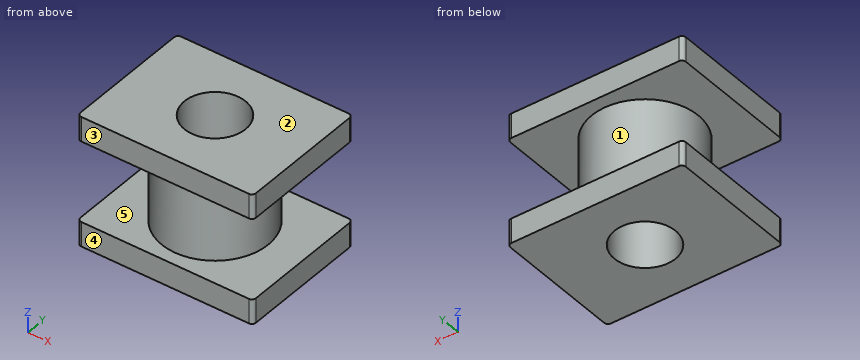
```python
from build123d import *

# Parameters (mm, degrees)
F0_R     = 2.7
F0_R_2   = 1.55
F1_DEPTH = 2.05
F2_W     = 8.9
F2_H     = 6.7
F2_R     = 2.7
F2_R_2   = 1.55
F3_DEPTH = 1.25
F4_R     = 0.2


with BuildPart() as f1:
    # F0 (on Top) → F1 (new body)
    with BuildSketch(Plane.XY):
        Circle(F0_R)
        Circle(F0_R_2, mode=Mode.SUBTRACT)
    extrude(amount=F1_DEPTH)

    # F2 (on face) → F3 (join)
    with BuildSketch(Plane.XY.offset(2.05)):
        Rectangle(F2_W, F2_H)
        Circle(F2_R, mode=Mode.SUBTRACT)
        Circle(F2_R)
        Circle(F2_R_2, mode=Mode.SUBTRACT)
    extrude(amount=F3_DEPTH)

    # F4
    f4_edges = [f1.edges().sort_by_distance(p)[0] for p in [
        (4.45, -3.35, 2.675),
        (-4.45, -3.35, 2.675),
        (-4.45, 3.35, 2.675),
        (4.45, 3.35, 2.675),
    ]]
    fillet(f4_edges, radius=F4_R)

    # F5: F1 across plane


with BuildPart() as f1_1:
    add(f1.part)
    add(f1.part.mirror(Plane.XY))


solid = f1_1.part
```
Here's how the part is built. I have some questions about the finished solid (model axes, mm). Face numbers are marked on the shaded views. A direction names the side the tool comes from. Give positions to 0.01 mm unless a question says otherwise; leave off trailing zeros. Loops run counter-clockwise (first coordinate to the right, second up) from the corner with the lowest first, then second, coordinate; pieces in that order, holes last. Notation, with made-up numbers: M 76,60.25 L 82,60.25 A18 ccw 82,66.25 Z; hole C 41,-16.75 d3. An arc over 180 degrees is marked long. Return JSON: item names as keys, results as strings.
Item 1: I'm going to push flat-ended pins straight in: pin 1 Ø2.5 at (x, y) = (0, 0) entering from +Z; pin 2 Ø3 at (x, z) = (0.5, 0) entering from -Y. Where does each tip first touch, or does it pass through?
A:
{"pin 1": "passes through", "pin 2": "stops at y = -2.7"}
Item 2: Thinking about a two-plate mould opening in Z: for the marked faces 1, 2 and 3, which applies, released by +Z, released by -Z, zero draft, split by the parting line, or undercut?
A:
{"face 1": "undercut", "face 2": "released by +Z", "face 3": "zero draft"}
Item 3: Imagine slicing it at B-B on x = 0. List the corners of the cut face in (y, z) for me, then the cut area to 3 significant figures.
A:
{"outline": "M -3.35,-3.3 L -1.55,-3.3 L -1.55,3.3 L -3.35,3.3 L -3.35,2.05 L -2.7,2.05 L -2.7,-2.05 L -3.35,-2.05 Z; M 1.55,-3.3 L 3.35,-3.3 L 3.35,-2.05 L 2.7,-2.05 L 2.7,2.05 L 3.35,2.05 L 3.35,3.3 L 1.55,3.3 Z", "area": "18.4 mm^2"}
Item 4: Please list where these lines run through material, in increasing order: line 1 (Z direction, x = -2.25, y = 2); line 2 (Y direction, x = 0, z = 1.5); line 3 (X direction, y = -0.5, z = 0.75).
A:
{"line 1": "z = -3.3 to -2.05, 2.05 to 3.3", "line 2": "y = -2.7 to -1.55, 1.55 to 2.7", "line 3": "x = -2.65 to -1.47, 1.47 to 2.65"}
Item 5: Imagine slicing it at D-D on x = -3. List the corners of the cut face in (y, z) for me.
A:
{"outline": "M -3.35,-3.3 L 3.35,-3.3 L 3.35,-2.05 L -3.35,-2.05 Z; M -3.35,2.05 L 3.35,2.05 L 3.35,3.3 L -3.35,3.3 Z"}
Item 6: Imagine slicing it at C-C on z = 0. List the corners of the cut face in (x, y) for me.
A:
{"outline": "C 0,0 d5.4; hole C 0,0 d3.1"}
Item 7: On a 3-axis mill with a long thin cutter (end or side, diameter ignored), from which of +Z, -Z, +X, -X, +Y, -Y can I reach the whole of each face in a straight line? I mean the marked faces 4 and 5. Say none if no direction works.
A:
{"face 4": "+Z, -Z, +X, -X, -Y", "face 5": "none"}
Item 8: Imagine slicing it at A-A on y = 0. List the corners of the cut face in (x, z) for me.
A:
{"outline": "M -4.45,-3.3 L -1.55,-3.3 L -1.55,3.3 L -4.45,3.3 L -4.45,2.05 L -2.7,2.05 L -2.7,-2.05 L -4.45,-2.05 Z; M 1.55,-3.3 L 4.45,-3.3 L 4.45,-2.05 L 2.7,-2.05 L 2.7,2.05 L 4.45,2.05 L 4.45,3.3 L 1.55,3.3 Z"}
